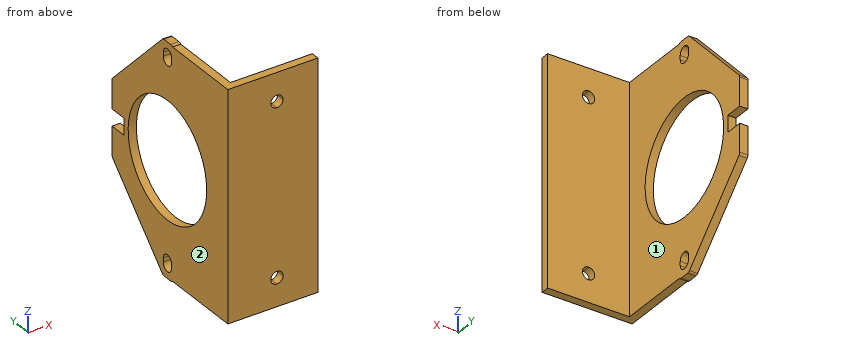
```python
from build123d import *

# Parameters (mm, degrees)
SKETCH1_R           = 14.2
SKETCH1_W           = 4.4
SKETCH1_H           = 4.2
BOSS_EXTRUDE1_DEPTH = 2
BOSS_EXTRUDE2_DEPTH = 2
SKETCH3_W           = 55.560809748
SKETCH3_H           = 2
BOSS_EXTRUDE3_DEPTH = 20
CUT_EXTRUDE1_DEPTH  = 2


with BuildPart() as part:
    # Sketch1 → Boss-Extrude1 (new body)
    with BuildSketch(Plane(origin=(668.139739498, 0, 0), x_dir=(0, 0, -1), z_dir=(1, 0, 0))):
        with BuildLine():
            ThreePointArc((-1314.332175016, 878.774707493), (-1314.042285701, 878.583942821), (-1313.701770142, 878.517038946))
            Line((-1313.701770142, 878.517038946), (-1306.83550516, 878.517038946))
            Line((-1306.83550516, 878.517038946), (-1306.83550516, 882.842038946))
            Line((-1306.83550516, 882.842038946), (-1302.78550516, 882.842038946))
            Line((-1302.78550516, 882.842038946), (-1302.78550516, 878.517038946))
            Line((-1302.78550516, 878.517038946), (-1295.919240178, 878.517038946))
            ThreePointArc((-1295.919240178, 878.517038946), (-1295.578724618, 878.583942821), (-1295.288835304, 878.774707493))
            Line((-1295.288835304, 878.774707493), (-1277.030100286, 896.694420906))
            ThreePointArc((-1277.030100286, 896.694420906), (-1276.830636379, 896.988445301), (-1276.76050516, 897.336752359))
            Line((-1276.76050516, 897.336752359), (-1276.76050516, 899.747325533))
            ThreePointArc((-1276.76050516, 899.747325533), (-1276.830636379, 900.095632591), (-1277.030100286, 900.389656986))
            Line((-1277.030100286, 900.389656986), (-1295.288835304, 918.309370399))
            ThreePointArc((-1295.288835304, 918.309370399), (-1295.578724618, 918.500135071), (-1295.919240178, 918.567038946))
            Line((-1295.919240178, 918.567038946), (-1302.78550516, 918.567038946))
            Line((-1302.78550516, 918.567038946), (-1302.78550516, 914.242038946))
            Line((-1302.78550516, 914.242038946), (-1306.83550516, 914.242038946))
            Line((-1306.83550516, 914.242038946), (-1306.83550516, 918.567038946))
            Line((-1306.83550516, 918.567038946), (-1313.701770142, 918.567038946))
            ThreePointArc((-1313.701770142, 918.567038946), (-1314.042285701, 918.500135071), (-1314.332175016, 918.309370399))
            Line((-1314.332175016, 918.309370399), (-1332.590910034, 900.389656986))
            ThreePointArc((-1332.590910034, 900.389656986), (-1332.79037394, 900.095632591), (-1332.86050516, 899.747325533))
            Line((-1332.86050516, 899.747325533), (-1332.86050516, 897.336752359))
            ThreePointArc((-1332.86050516, 897.336752359), (-1332.79037394, 896.988445301), (-1332.590910034, 896.694420906))
            Line((-1332.590910034, 896.694420906), (-1314.332175016, 878.774707493))
        make_face()
        with Locations((-1304.81050516, 898.542038946)):
            Circle(SKETCH1_R, mode=Mode.SUBTRACT)
        with BuildLine():
            Line((-1329.71050516, 900.042038946), (-1328.71050516, 900.042038946))
            ThreePointArc((-1328.71050516, 900.042038946), (-1327.21050516, 898.542038946), (-1328.71050516, 897.042038946))
            Line((-1328.71050516, 897.042038946), (-1329.71050516, 897.042038946))
            ThreePointArc((-1329.71050516, 897.042038946), (-1330.771165332, 897.481378774), (-1331.21050516, 898.542038946))
            ThreePointArc((-1331.21050516, 898.542038946), (-1330.771165332, 899.602699118), (-1329.71050516, 900.042038946))
        make_face(mode=Mode.SUBTRACT)
        with BuildLine():
            ThreePointArc((-1279.91050516, 900.042038946), (-1278.41050516, 898.542038946), (-1279.91050516, 897.042038946))
            Line((-1279.91050516, 897.042038946), (-1280.91050516, 897.042038946))
            ThreePointArc((-1280.91050516, 897.042038946), (-1281.971165332, 897.481378774), (-1282.41050516, 898.542038946))
            ThreePointArc((-1282.41050516, 898.542038946), (-1281.971165332, 899.602699118), (-1280.91050516, 900.042038946))
            Line((-1280.91050516, 900.042038946), (-1279.91050516, 900.042038946))
        make_face(mode=Mode.SUBTRACT)
        with Locations((-1286.76050516, 898.542038946)):
            Rectangle(SKETCH1_W, SKETCH1_H, mode=Mode.SUBTRACT)
        with Locations((-1322.86050516, 898.542038946)):
            Rectangle(SKETCH1_W, SKETCH1_H, mode=Mode.SUBTRACT)
        with Locations((-1322.86050516, 898.542038946)):
            Rectangle(SKETCH1_W, SKETCH1_H)
        with Locations((-1286.76050516, 898.542038946)):
            Rectangle(SKETCH1_W, SKETCH1_H)
    extrude(amount=BOSS_EXTRUDE1_DEPTH)

    # Sketch2 → Boss-Extrude2 (add)
    with BuildSketch(Plane(origin=(670.139739498, 0, 0), x_dir=(0, 0, -1), z_dir=(1, 0, 0))):
        with BuildLine():
            Line((-1332.590910034, 876.694420906), (-1277.030100286, 876.694420906))
            Line((-1277.030100286, 876.694420906), (-1277.030100286, 896.694420906))
            Line((-1277.030100286, 896.694420906), (-1295.288835304, 878.774707493))
            ThreePointArc((-1295.288835304, 878.774707493), (-1295.578724618, 878.583942821), (-1295.919240178, 878.517038946))
            Line((-1295.919240178, 878.517038946), (-1302.78550516, 878.517038946))
            Line((-1302.78550516, 878.517038946), (-1302.78550516, 882.842038946))
            Line((-1302.78550516, 882.842038946), (-1306.83550516, 882.842038946))
            Line((-1306.83550516, 882.842038946), (-1306.83550516, 878.517038946))
            Line((-1306.83550516, 878.517038946), (-1313.701770142, 878.517038946))
            ThreePointArc((-1313.701770142, 878.517038946), (-1314.042285701, 878.583942821), (-1314.332175016, 878.774707493))
            Line((-1314.332175016, 878.774707493), (-1332.590910034, 896.694420906))
            Line((-1332.590910034, 896.694420906), (-1332.590910034, 876.694420906))
        make_face()
    extrude(amount=-BOSS_EXTRUDE2_DEPTH)

    # Sketch3 → Boss-Extrude3 (add)
    with BuildSketch(Plane(origin=(670.139739498, 0, 0), x_dir=(0, 0, -1), z_dir=(1, 0, 0))):
        with Locations((-1304.81050516, 877.694420906)):
            Rectangle(SKETCH3_W, SKETCH3_H)
    extrude(amount=BOSS_EXTRUDE3_DEPTH)

    # Sketch4 → Cut-Extrude1 (cut)
    with BuildSketch(Plane(origin=(0, 878.694420906, 0), x_dir=(1, 0, 0), z_dir=(0, 1, 0))):
        with BuildLine():
            ThreePointArc((681.639739498, -1283.920302723), (681.20039967, -1282.859642551), (680.139739498, -1282.420302723))
            Line((680.139739498, -1282.420302723), (680.139739498, -1285.420302723))
            ThreePointArc((680.139739498, -1285.420302723), (681.20039967, -1284.980962895), (681.639739498, -1283.920302723))
        make_face()
        with BuildLine():
            Line((680.139739498, -1285.420302723), (680.139739498, -1282.420302723))
            ThreePointArc((680.139739498, -1282.420302723), (678.639739498, -1283.920302723), (680.139739498, -1285.420302723))
        make_face()
        with BuildLine():
            ThreePointArc((681.639739498, -1325.700707597), (681.20039967, -1324.640047425), (680.139739498, -1324.200707597))
            Line((680.139739498, -1324.200707597), (680.139739498, -1327.200707597))
            ThreePointArc((680.139739498, -1327.200707597), (681.20039967, -1326.761367768), (681.639739498, -1325.700707597))
        make_face()
        with BuildLine():
            Line((680.139739498, -1327.200707597), (680.139739498, -1324.200707597))
            ThreePointArc((680.139739498, -1324.200707597), (678.639739498, -1325.700707597), (680.139739498, -1327.200707597))
        make_face()
    extrude(amount=-CUT_EXTRUDE1_DEPTH, mode=Mode.SUBTRACT)


solid = part.part
```
Could you check a few things on this model? Use its own coordinates, in mm. Face numbers are marked on the shaded views. A direction names the side the tool comes from. Give positions to 0.01 mm unless a question says otherwise; leave off trailing zeros. Loops run counter-clockwise (first coordinate to the right, second up) from the corner with the lowest first, then second, coordinate; pieces in that order, holes last. Notation, with made-up numbers: (32.25, 15.25) - (72.25, 15.25) arc R27 cw to (72.25, 37.25) - close; hole circle Ø7 at (4.5, 35). An arc over 180 degrees is marked (long way). Answer in a Markdown table with one row per item. Add a question column.
Q1. Please list where these lines run through material, in increasing order: L1, parallel to Y at x = 670.75, z = 1281; L2, parallel to X at y = 887, z = 1281; L3, parallel to Y at x = 669, z = 1296.5. Write a range as from..to.
Q2. If we section it at D-D (y = 903): List the corners of the cut face in (x, z) for me.
Q3. If we section it at A-A (z = 1291.5): List the corners of the cut face in (x, y) for me.
Q4. Which directions (+Z, -Z, +X, -X, +Y, -Y) give clear straight access to the entire face, cutting with the end or side of a thin tool? Please do the marked faces 1 and 2.
Q5. If we section it at B-B (y = 907.5): List the corners of the cut face in (x, z) for me, plus the area to 3 significant figures.
Q6. If we section it at C-C (x = 677.25): List the corners of the cut face in (y, z) for me.
Q7. For pin 1 (0.6 mm diameter, centred on x = 668.5, y = 916, fed in from +Z); pin 2 (0.8 mm diameter, centred on x = 669.5, z = 1280.5, fed in from +Y); pin 3 (12 mm diameter, centred on y = 900, z = 1307, fed in from +X); pin 4 (1 mm diameter, centred on x = 669.5, y = 915.5, fed in from -Z), each with a flat end and sliding along its axis, tell me the tip position at first contact or that it passes through.
The answers:
| question | item | result |
|---|---|---|
| 1 | L1 | y = 876.69..878.69 |
| 1 | L2 | x = 668.14..670.14 |
| 1 | L3 | y = 876.69..887.03, 910.06..918.57 |
| 2 | outline | (668.14, 1279.69) - (670.14, 1279.69) - (670.14, 1291.33) - (668.14, 1291.33) - close; (668.14, 1318.29) - (670.14, 1318.29) - (670.14, 1329.93) - (668.14, 1329.93) - close |
| 3 | outline | (668.14, 876.69) - (690.14, 876.69) - (690.14, 878.69) - (670.14, 878.69) - (670.14, 893.6) - (668.14, 893.6) - close; (668.14, 903.49) - (670.14, 903.49) - (670.14, 914.59) - (668.14, 914.59) - close |
| 4 | face 1 | +Z, -Z, +X, +Y |
| 4 | face 2 | +Z, -Z, -X, +Y, -Y |
| 5 | outline | (668.14, 1284.27) - (670.14, 1284.27) - (670.14, 1293.79) - (668.14, 1293.79) - close; (668.14, 1315.83) - (670.14, 1315.83) - (670.14, 1325.35) - (668.14, 1325.35) - close |
| 5 | area | 38.1 mm^2 |
| 6 | outline | (876.69, 1277.03) - (878.69, 1277.03) - (878.69, 1332.59) - (876.69, 1332.59) - close |
| 7 | pin 1 | stops at z = 1316.99 |
| 7 | pin 2 | stops at y = 904.19 |
| 7 | pin 3 | passes through |
| 7 | pin 4 | stops at z = 1291.92 |
